```python
from build123d import *

# Parameters (mm, degrees)
SKETCH1_R           = 66.675
BOSS_EXTRUDE1_DEPTH = 6.35
CUT_EXTRUDE1_DEPTH  = 7.35


with BuildPart() as part:
    # Sketch1 → Boss-Extrude1 (new body)
    with BuildSketch(Plane.XY):
        Circle(SKETCH1_R)
    extrude(amount=BOSS_EXTRUDE1_DEPTH)

    # Sketch2 → Cut-Extrude1 (cut, through all)
    with BuildSketch(Plane.XY.offset(6.35)):
        Polygon((-40.005, 0), (-40.005, 3.175), (-67.945, 3.175), (-67.945, -3.175), (-40.005, -3.175), align=None)
        Polygon((40.005, -3.175), (40.005, 0), (40.005, 3.175), (67.945, 3.175), (67.945, -3.175), align=None)
    extrude(amount=-CUT_EXTRUDE1_DEPTH, mode=Mode.SUBTRACT)


solid = part.part
```
Source: CAD feature listing. Evaluate the final solid. Frame: model axes, mm. A direction names the side the tool comes from. Coordinates: 2 decimals unless noted, no trailing zeros. Loops run counter-clockwise (first coordinate to the right, second up) from the corner with the lowest first, then second, coordinate; pieces in that order, holes last. Notation, with made-up numbers: (-17.75, -10) - (25.25, -10) arc R23 cw to (25.25, 5) - close; hole circle Ø4 at (69, -4.5). An arc over 180 degrees is marked (long way). Answer as CSV lines item,"result".
1. Section D-D (x = 15.5). Return loops of the section in (y, z).
Established:
outline,"(-64.85, 0) - (64.85, 0) - (64.85, 6.35) - (-64.85, 6.35) - close"
2. Reachability of faces 1 (the flat face through (-1, 1, 0)), 2 (the flat face through (53, 3.175, 3)), 3 (the flat face through (-53, 3.175, 3)) from +Z, -Z, +X, -X, +Y, -Y: full face, straight path, thin tool, end or side. Return the list, or none.
Established:
face 1,"-Z, +X, -X, +Y, -Y"
face 2,"+Z, -Z, +X"
face 3,"+Z, -Z, -X"
3. Mould query, pull axis Y, two halves, no side actions, for faces 4 (the flat face through (-53, -3.175, 3)), 5 (the flat face through (-1, 1, 6.35)), 6 (the flat face through (-40.005, 0, 3)), 7 (the cylindrical face through (1.42, 66.66, 3.13)). Classes: released by +Y, released by -Y, zero draft, split by the parting line, or undercut.
Established:
face 4,"undercut"
face 5,"zero draft"
face 6,"undercut"
face 7,"released by +Y"
4. Ray query, line 1 (Y direction, x = 42.5, z = 5.25) (3 decimals); line 2 (Y direction, x = -50.5, z = 1.5) (3 decimals); line 3 (Y direction, x = -3.5, z = 5). Return the intervals inside material, ascending.
Established:
line 1,"y = -51.374 to -3.175, 3.175 to 51.374"
line 2,"y = -43.535 to -3.175, 3.175 to 43.535"
line 3,"y = -66.58 to 66.58"
5. Section A-A (z = 4.25). Return loops of the section in (x, y) (3 decimals).
Established:
outline,"(-66.599, -3.175) arc R66.675 ccw to (66.599, -3.175) - (40.005, -3.175) - (40.005, 3.175) - (66.599, 3.175) arc R66.675 ccw to (-66.599, 3.175) - (-40.005, 3.175) - (-40.005, -3.175) - close"
6. Section B-B (x = 53.5). Return loops of the section in (y, z) (3 decimals), then the cut area to 3 significant figures.
Established:
outline,"(-39.791, 0) - (-3.175, 0) - (-3.175, 6.35) - (-39.791, 6.35) - close; (3.175, 0) - (39.791, 0) - (39.791, 6.35) - (3.175, 6.35) - close"
area,"465 mm2"
7. Section C-C (y = 0). Return loops of the section in (x, z) (3 decimals), then the cut area to 3 significant figures.
Established:
outline,"(-40.005, 0) - (40.005, 0) - (40.005, 6.35) - (-40.005, 6.35) - close"
area,"508 mm2"
8. Contact query for flat-ended pins moving along their axis: pin 1 (1.9 mm diameter, centred on x = 59.5, z = 3, fed in from +Y); pin 2 (3 mm diameter, centred on x = -48, z = 4, fed in from +Y). Output: stop coordinate, or through.
Established:
pin 1,"stops at y = 31.9"
pin 2,"stops at y = 47.78"
